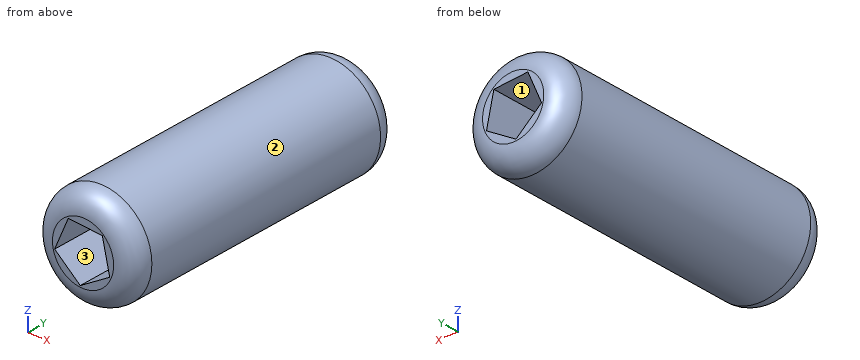
from build123d import *

# Parameters (mm, degrees)
F0_R     = 12.400865
F1_DEPTH = 75.2
F2_R     = 5
F4_DEPTH = 95


with BuildPart() as f1:
    # F0 (on Front) → F1 (new body)
    with BuildSketch(Plane.XZ):
        Circle(F0_R)
    extrude(amount=F1_DEPTH)

    # F2
    f2_edges = [f1.edges().sort_by_distance(p)[0] for p in [
        (-12.400865, -75.2, 0),
        (12.400865, -37.6, 0),
        (-12.400865, 0, 0),
    ]]
    fillet(f2_edges, radius=F2_R)

    # F3 (on Front) → F4 (cut)
    with BuildSketch(Plane.XZ):
        Polygon((-0.678238, -6.999642), (6.447468, -2.808051), (4.662992, 5.264171), (-3.56558, 6.061488), (-6.866642, -1.517966), align=None)
    extrude(amount=F4_DEPTH, mode=Mode.SUBTRACT)


solid = f1.part
Could you check a few things on this model? Use its own coordinates, in mm. Face numbers are marked on the shaded views. Give positions to 0.01 mm unless a question says otherwise; leave off trailing zeros. Loops run counter-clockwise (first coordinate to the right, second up) from the corner with the lowest first, then second, coordinate; pieces in that order, holes last. Notation, with made-up numbers: (29.5, 11) -> (75.5, 11) arc R18 ccw to (75.5, 26) -> close; hole circle Ø8 at (3.25, 24.5). An arc over 180 degrees is marked (long way). Return JSON: item names as keys, results as strings.
Item 1: If we section it at C-C on x = 0: List the corners of the cut face in (y, z) for me.
Geometry results:
{"outline": "(-75.2, -7.4) arc R5 ccw to (-70.2, -12.4) -> (-5, -12.4) arc R5 ccw to (0, -7.4) -> (0, -6.6) -> (-75.2, -6.6) -> close; (-75.2, 5.72) -> (0, 5.72) -> (0, 7.4) arc R5 ccw to (-5, 12.4) -> (-70.2, 12.4) arc R5 ccw to (-75.2, 7.4) -> close"}
Item 2: We'd pull the mould along Z, two halves only. Please class the marked faces 1, 2 and 3: +Z half, -Z half, draft (parallel to the pull), parting line (faces both ways), or undercut.
Geometry results:
{"face 1": "undercut", "face 2": "parting line", "face 3": "undercut"}
Item 3: If we section it at A-A on y = -29.5: List the corners of the cut face in (x, z) for me, plus the area to 3 significant figures.
Geometry results:
{"outline": "circle Ø24.8 at (0, 0); hole (-6.87, -1.52) -> (-0.68, -7) -> (6.45, -2.81) -> (4.66, 5.26) -> (-3.57, 6.06) -> close", "area": "366 mm²"}
Item 4: I need wall thicknesses on L1, parallel to Z at x = 0.75, y = -56.5; L2, parallel to X at y = -10, z = 3; L3, parallel to Z at x = 2.5, y = -4. Which ranges of each line are inside material? Lowest first, please. Write a range as from..to.
Geometry results:
{"L1": "z = -12.38..-6.16, 5.64..12.38", "L2": "x = -12.03..-4.9, 5.16..12.03", "L3": "z = -12.04..-5.13, 5.47..12.04"}
Item 5: I'm going to push flat-ended pins straight in: pin 1 (12 mm diameter, centred on y = -51, z = 8.5, fed in from -X); pin 2 (1 mm diameter, centred on y = -64, z = 4, fed in from -X); pin 3 (1.5 mm diameter, centred on x = -7, z = 9, fed in from -Y). Where does each tip first touch, or does it pass through?
Geometry results:
{"pin 1": "stops at x = -12.15", "pin 2": "stops at x = -11.9", "pin 3": "stops at y = -74"}
Item 6: If we section it at B-B on z = 0: List the corners of the cut face in (x, y) for me, plus the area to 3 significant figures.
Geometry results:
{"outline": "(-12.4, -70.2) arc R5 ccw to (-7.4, -75.2) -> (-6.21, -75.2) -> (-6.21, 0) -> (-7.4, 0) arc R5 ccw to (-12.4, -5) -> close; (5.83, -75.2) -> (7.4, -75.2) arc R5 ccw to (12.4, -70.2) -> (12.4, -5) arc R5 ccw to (7.4, 0) -> (5.83, 0) -> close", "area": "939 mm²"}
